Design review of the part built by this model. Coordinates are the model's own, in mm. Give positions to 0.01 mm unless a question says otherwise; leave off trailing zeros. Write each loop counter-clockwise with the first axis right and the second up, starting at its lowest first coordinate (ties: lowest second). Pieces come first, ordered by that corner, then holes. Notation, with made-up numbers: (24, 39.25) -> (60, 39.25) arc R20 cw to (60, 55.25) -> close; hole circle Ø2 at (17, 77.5). An arc over 180 degrees is marked (long way). Write each question's results on one line, items separated by ' | '. Start each with the question number.
(1) To check wall thickness, follow probe 1 along Y at (x, z) = (35, 38.5); probe 2 along X at (y, z) = (45, 27); probe 3 along Y at (x, z) = (35.5, 15.5). State the ranges of each line that lie inside material, in increasing order.
(2) Take a section at A-A (y = 45). State the section outline as (x, z) points, plus the area to 3 significant figures.
(3) Take a section at B-B (x = 35). State the section outline as (y, z) points.
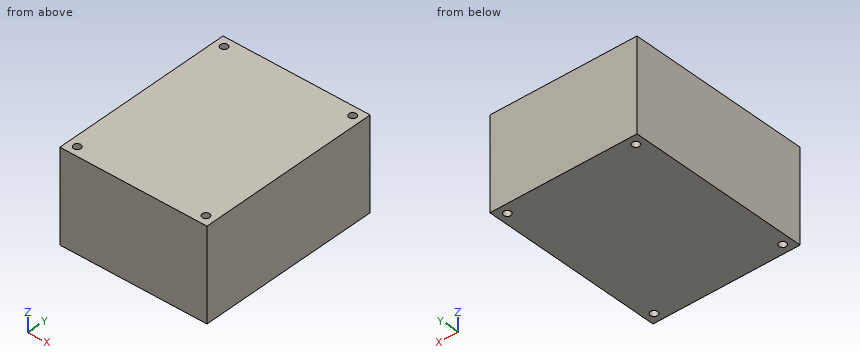
Autodesk Inventor part; units mm, degrees
sketch "Sketch2" plane through (0, 0, 0) normal (0, 0, 1) x (1, 0, 0)
  line L0 (40, -50) -> (-40, -50)
  line L1 (-40, -50) -> (-40, 50)
  line L2 (-40, 50) -> (40, 50)
  line L3 (40, 50) -> (40, -50)
  line L4 (40, -50) -> (-40, 50) construction
  line L5 (-40, -50) -> (40, 50) construction
  point P0 (0, 0)
  dimension "d0" = 100
  dimension "d1" = 80
extrude "Extrusion1" add sketch "Sketch2" along normal blind 50
sketch "Sketch3" plane through (0, 0, 50) normal (0, 0, 1) x (1, 0, 0)
  line L0 (40, 50) -> (-40, 50) construction
  line L1 (-40, 50) -> (-40, -50) construction
  line L2 (-40, -50) -> (40, -50) construction
  line L3 (40, -50) -> (40, 50) construction
  point P0 (0, 0)
  point P1 (-35, 45)
  point P2 (35, 45)
  point P3 (-35, -45)
  point P4 (35, -45)
  dimension "d4" = 5
  dimension "d5" = 5
  dimension "d6" = 5
  dimension "d7" = 5
  dimension "d8" = 5
  dimension "d9" = 5
  dimension "d10" = 5
  dimension "d11" = 5
hole "Hole1" at (-35, 45, 50) at (35, 45, 50) at (-35, -45, 50) at (35, -45, 50) direction (0, 0, -1) diameter 4 depth 50
properties part number "P028_PCB_surMesures"
Report:
1) probe 1: -50 to -47, -43 to 43, 47 to 50 | probe 2: -40 to -37, -33 to 33, 37 to 40 | probe 3: -50 to -46.94, -43.06 to 43.06, 46.94 to 50
2) outline: (-40, 0) -> (-37, 0) -> (-37, 50) -> (-40, 50) -> close; (-33, 0) -> (33, 0) -> (33, 50) -> (-33, 50) -> close; (37, 0) -> (40, 0) -> (40, 50) -> (37, 50) -> close | area: 3,600 mm2
3) outline: (-50, 0) -> (-47, 0) -> (-47, 50) -> (-50, 50) -> close; (-43, 0) -> (43, 0) -> (43, 50) -> (-43, 50) -> close; (47, 0) -> (50, 0) -> (50, 50) -> (47, 50) -> close
